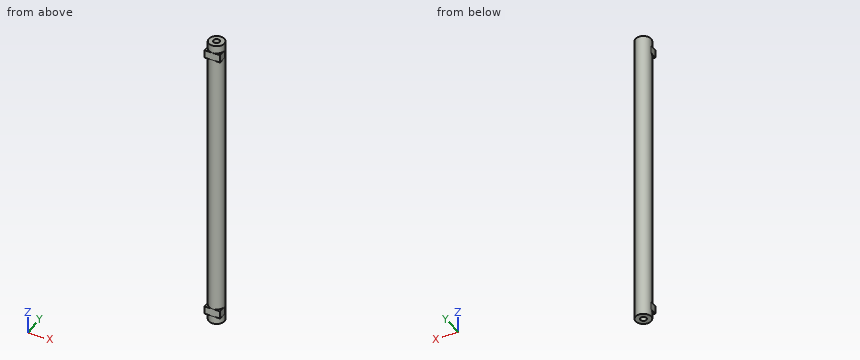
```python
from build123d import *

# Parameters (mm, degrees)
CYLINDER006_R     = 5
CYLINDER006_DEPTH = 192
BOX003_W          = 10
BOX003_H          = 5
BOX003_DEPTH      = 5
BOX004_W          = 10
BOX004_H          = 5
BOX004_DEPTH      = 5
CYLINDER007_R     = 2
CYLINDER007_DEPTH = 10
CYLINDER008_R     = 2
CYLINDER008_DEPTH = 10


with BuildPart() as part:
    # Cylinder006 → Cylinder006 (join)
    with BuildSketch(Plane.XY):
        Circle(CYLINDER006_R)
    extrude(amount=CYLINDER006_DEPTH)

    # Box003 → Box003 (join)
    with BuildSketch(Plane(origin=(-5, -5, 182), x_dir=(1, 0, 0), z_dir=(0, 0, 1))):
        with Locations((5, 2.5)):
            Rectangle(BOX003_W, BOX003_H)
    extrude(amount=BOX003_DEPTH)

    # Box004 → Box004 (join)
    with BuildSketch(Plane(origin=(-5, -5, 5), x_dir=(1, 0, 0), z_dir=(0, 0, 1))):
        with Locations((5, 2.5)):
            Rectangle(BOX004_W, BOX004_H)
    extrude(amount=BOX004_DEPTH)

    # Cylinder007 → Cylinder007 (cut)
    with BuildSketch(Plane.XY):
        Circle(CYLINDER007_R)
    extrude(amount=CYLINDER007_DEPTH, mode=Mode.SUBTRACT)

    # Cylinder008 → Cylinder008 (cut)
    with BuildSketch(Plane.XY.offset(182)):
        Circle(CYLINDER008_R)
    extrude(amount=CYLINDER008_DEPTH, mode=Mode.SUBTRACT)


with BuildPart() as part_1:
    # Body004 placement: moved
    add(part.part.moved(Location((1, -43, -192))))


solid = part_1.part
```
Could you check a few things on this model? Use its own coordinates, in mm. Round coordinates to 2 decimals unless told otherwise and drop trailing zeros. Order: outer loops, then holes, each group sorted by start corner. A loop starts at its lowest first (then second) coordinate and runs counter-clockwise, first axis right, second up. Notation, with made-up numbers: (-0.75, 44.5) -> (3.25, 44.5) arc R11 ccw to (3.25, 62.5) -> close; hole circle Ø3 at (5, -7.75). An arc over 180 degrees is marked (long way). One line per question, with ' | ' between items.
Q1. I'm going to push flat-ended pins straight in: pin 1 (1.2 mm diameter, centred on x = 0, y = -43.5, fed in from -Z); pin 2 (1 mm diameter, centred on y = -41, z = -51, fed in from +X); pin 3 (1.2 mm diameter, centred on x = 1.5, y = -43.5, fed in from +Z). Where does each tip first touch, or does it pass through?
Computed values:
pin 1: z = -182 | pin 2: x = 5.77 | pin 3: z = -10
Q2. If we section it at A-A on z = -18: Write out the boundary of the cut face in (x, y), plus the area to 3 significant figures.
Computed values:
outline: circle Ø10 at (1, -43) | area: 78.5 mm²
Q3. If we section it at B-B on y = -39.5: Write out the boundary of the cut face in (x, z).
Computed values:
outline: (-2.57, -192) -> (4.57, -192) -> (4.57, 0) -> (-2.57, 0) -> close
Q4. If I drill on line 1 (Y direction, x = 1, z = -187.25); line 2 (Z direction, x = -3, y = -46.5); line 3 (Y direction, x = 0.5, z = -56), over which ranges is the centre line in solid material (lowest first)? Write a range as from..to.
Computed values:
line 1: -48..-45, -41..-38 | line 2: -187..-182, -10..-5 | line 3: -47.97..-38.03
